Source: CAD feature listing. Evaluate the final solid. Frame: model axes, mm. A direction names the side the tool comes from. Coordinates: 2 decimals unless noted, no trailing zeros. Order: outer loops, then holes, each group sorted by start corner. A loop starts at its lowest first (then second) coordinate and runs counter-clockwise, first axis right, second up. Notation, with made-up numbers: (78, 51) -> (129, 51) arc R12 cw to (129, 67) -> close; hole circle Ø3 at (84.25, -7). An arc over 180 degrees is marked (long way). Write item = value, one per line. Start each with the question number.
Item 1: Section query A-A (y = 0). Output: boundary loops of the cut face in (x, z), then the cut area to 3 significant figures.
Item 2: Contact query for flat-ended pins moving along their axis: pin 1 (3.5 mm diameter, centred on x = 0, y = 0, fed in from -Z); pin 2 (5.5 mm diameter, centred on x = 0, y = 0, fed in from -Z). Output: stop coordinate, or through.
Item 3: Set-up query: faces 4 (the cylindrical face through (-1.825, -1.4, 1.972)), 5 (the flat face through (2, -5, 5)). Return all of +Z, -Z, +X, -X, +Y, -Y with unobstructed straight access to the full face (end or side cutting, diameter ignored); none if empty.
Item 4: Section query C-C (z = 1). Output: boundary loops of the cut face in (x, y).
Item 5: Ray query, line 1 along Y through (x, z) = (0, 0.9); line 2 along X through (y, z) = (0, 7.65); line 3 along Y through (x, z) = (0, 6.5). Return the intervals inside material, ascending. Write a range as [from, to].
Item 6: Section query B-B (x = 0). Output: boundary loops of the cut face in (y, z), then the cut area to 3 significant figures.
Item 7: Section query D-D (y = 21). Output: boundary loops of the cut face in (x, z).
Item 8: Mould query, pull axis X, two halves, no side actions, for faces 1 (the cylindrical face through (-0.37, -1.66, 6.96)), 2 (the flat face through (2, 10, 0)), 3 (the flat face through (-5, 10, 5)). Classes: released by +X, released by -X, zero draft, split by the parting line, or undercut.
```python
from build123d import *

# Parameters (mm, degrees)
CYLINDER002_R     = 1.8
CYLINDER002_DEPTH = 20
CYLINDER001_R     = 2.3
CYLINDER001_DEPTH = 10
CYLINDER_R        = 1.7
CYLINDER_DEPTH    = 10
BOX_W             = 15
BOX_H             = 30
BOX_DEPTH         = 10


with BuildPart() as m3_clear:
    # Cylinder002 → Cylinder002 (new body)
    with BuildSketch(Plane(origin=(0, 21, -4), x_dir=(1, 0, 0), z_dir=(0, 0, 1))):
        Circle(CYLINDER002_R)
    extrude(amount=CYLINDER002_DEPTH)


with BuildPart() as cylinder001:
    # Cylinder001 → Cylinder001 (new body)
    with BuildSketch(Plane.XY):
        Circle(CYLINDER001_R)
    extrude(amount=CYLINDER001_DEPTH)


with BuildPart() as fusion001:
    # Cylinder → Cylinder (new body)
    with BuildSketch(Plane.XY.offset(7)):
        Circle(CYLINDER_R)
    extrude(amount=CYLINDER_DEPTH)

    # Fusion: union Cylinder001
    add(cylinder001.part)


with BuildPart() as fusion001_1:
    # Fusion placement: moved
    add(fusion001.part.moved(Location((0, 0, -6))))

    # Fusion001: union M3-clear
    add(m3_clear.part)


with BuildPart() as cut:
    # Box → Box (new body)
    with BuildSketch(Plane(origin=(-5, -5, 0), x_dir=(1, 0, 0), z_dir=(0, 0, 1))):
        with Locations((7.5, 15)):
            Rectangle(BOX_W, BOX_H)
    extrude(amount=BOX_DEPTH)

    # Cut: cut Fusion001
    add(fusion001_1.part, mode=Mode.SUBTRACT)


solid = cut.part
```
Computed:
q1.outline = (-5, 0) -> (-2.3, 0) -> (-2.3, 4) -> (-1.7, 4) -> (-1.7, 10) -> (-5, 10) -> close; (1.7, 4) -> (2.3, 4) -> (2.3, 0) -> (10, 0) -> (10, 10) -> (1.7, 10) -> close
q1.area = 111 mm^2
q2.pin_1 = 4
q2.pin_2 = 0
q3.face_4 = -Z
q3.face_5 = +Z, -Z, +X, -X, -Y
q4.outline = (-5, -5) -> (10, -5) -> (10, 25) -> (-5, 25) -> close; hole circle Ø4.6 at (0, 0); hole circle Ø3.6 at (0, 21)
q5.line_1 = [-5, -2.3], [2.3, 19.2], [22.8, 25]
q5.line_2 = [-5, -1.7], [1.7, 10]
q5.line_3 = [-5, -1.7], [1.7, 19.2], [22.8, 25]
q6.outline = (-5, 0) -> (-2.3, 0) -> (-2.3, 4) -> (-1.7, 4) -> (-1.7, 10) -> (-5, 10) -> close; (1.7, 4) -> (2.3, 4) -> (2.3, 0) -> (19.2, 0) -> (19.2, 10) -> (1.7, 10) -> close; (22.8, 0) -> (25, 0) -> (25, 10) -> (22.8, 10) -> close
q6.area = 225 mm^2
q7.outline = (-5, 0) -> (-1.8, 0) -> (-1.8, 10) -> (-5, 10) -> close; (1.8, 0) -> (10, 0) -> (10, 10) -> (1.8, 10) -> close
q8.face_1 = undercut
q8.face_2 = zero draft
q8.face_3 = released by -X
